from build123d import *

# Parameters (mm, degrees)
SKETCH1_R           = 6.35
BOSS_EXTRUDE1_DEPTH = 2.54
BOSS_EXTRUDE2_DEPTH = 12.7
SKETCH2_3_R         = 12.7
SKETCH2_3_R_2       = 6.35
BOSS_EXTRUDE3_DEPTH = 19.05
SKETCH2_5_R         = 6.35
BOSS_EXTRUDE4_DEPTH = 7.62
SKETCH5_R           = 6.35
CUT_EXTRUDE1_DEPTH  = 7.62


with BuildPart() as part:
    # Sketch1 → Boss-Extrude1 (new body)
    with BuildSketch(Plane(origin=(0, 0, 0), x_dir=(1, 0, 0), z_dir=(0, 1, 0))):
        with BuildLine():
            Line((12.7, 0), (63.5, 0))
            ThreePointArc((63.5, 0), (72.480256121, 3.719743879), (76.2, 12.7))
            Line((76.2, 12.7), (76.2, 50.8))
            ThreePointArc((76.2, 50.8), (72.480256121, 59.780256121), (63.5, 63.5))
            Line((63.5, 63.5), (12.7, 63.5))
            ThreePointArc((12.7, 63.5), (3.719743879, 59.780256121), (0, 50.8))
            Line((0, 50.8), (0, 12.7))
            ThreePointArc((0, 12.7), (3.719743879, 3.719743879), (12.7, 0))
        make_face()
        with Locations((12.7, 12.7)):
            Circle(SKETCH1_R, mode=Mode.SUBTRACT)
        with Locations((63.5, 12.7)):
            Circle(SKETCH1_R, mode=Mode.SUBTRACT)
    extrude(amount=BOSS_EXTRUDE1_DEPTH)

    # Sketch2 → Boss-Extrude2 (add)
    with BuildSketch(Plane(origin=(0, 2.54, 0), x_dir=(1, 0, 0), z_dir=(0, 1, 0))):
        with BuildLine():
            Line((63.5, 63.5), (12.7, 63.5))
            ThreePointArc((12.7, 63.5), (3.719743879, 59.780256121), (0, 50.8))
            ThreePointArc((0, 50.8), (0.544931264, 47.119741312), (2.132961262, 43.755307508))
            Line((2.132961262, 43.755307508), (27.532961262, 5.655307508))
            ThreePointArc((27.532961262, 5.655307508), (34.419741312, 24.855068736), (50.8, 12.7))
            ThreePointArc((50.8, 12.7), (50.255068736, 9.019741312), (48.667038738, 5.655307508))
            Line((48.667038738, 5.655307508), (74.067038738, 43.755307508))
            ThreePointArc((74.067038738, 43.755307508), (75.655068736, 47.119741312), (76.2, 50.8))
            ThreePointArc((76.2, 50.8), (72.480256121, 59.780256121), (63.5, 63.5))
        make_face()
        with BuildLine():
            Line((23.553103988, 16.204143539), (5.488594295, 43.300908078))
            ThreePointArc((5.488594295, 43.300908078), (4.924935684, 54.961088143), (14.939453481, 60.96))
            Line((14.939453481, 60.96), (61.260546519, 60.96))
            ThreePointArc((61.260546519, 60.96), (71.275064316, 54.961088143), (70.711405705, 43.300908078))
            Line((70.711405705, 43.300908078), (52.646896012, 16.204143539))
            ThreePointArc((52.646896012, 16.204143539), (38.1, 27.662994537), (23.553103988, 16.204143539))
        make_face(mode=Mode.SUBTRACT)
    extrude(amount=BOSS_EXTRUDE2_DEPTH)

    # Sketch2_3 → Boss-Extrude3 (add)
    with BuildSketch(Plane(origin=(0, 2.54, 0), x_dir=(1, 0, 0), z_dir=(0, 1, 0))):
        with Locations((38.1, 12.7)):
            Circle(SKETCH2_3_R)
        with Locations((38.1, 12.7)):
            Circle(SKETCH2_3_R_2, mode=Mode.SUBTRACT)
    extrude(amount=BOSS_EXTRUDE3_DEPTH)

    # Sketch2_5 → Boss-Extrude4 (add)
    with BuildSketch(Plane(origin=(0, 2.54, 0), x_dir=(1, 0, 0), z_dir=(0, 1, 0))):
        with BuildLine():
            ThreePointArc((61.260546519, 60.96), (71.275064316, 54.961088143), (70.711405705, 43.300908078))
            Line((70.711405705, 43.300908078), (52.646896012, 16.204143539))
            ThreePointArc((52.646896012, 16.204143539), (38.1, 27.662994537), (23.553103988, 16.204143539))
            Line((23.553103988, 16.204143539), (5.488594295, 43.300908078))
            ThreePointArc((5.488594295, 43.300908078), (4.924935684, 54.961088143), (14.939453481, 60.96))
            Line((14.939453481, 60.96), (61.260546519, 60.96))
        make_face()
        with Locations((63.5, 50.8)):
            Circle(SKETCH2_5_R, mode=Mode.SUBTRACT)
        with Locations((12.7, 50.8)):
            Circle(SKETCH2_5_R, mode=Mode.SUBTRACT)
    extrude(amount=BOSS_EXTRUDE4_DEPTH)

    # Sketch5 → Cut-Extrude1 (cut)
    with BuildSketch(Plane(origin=(0, 2.54, 0), x_dir=(1, 0, 0), z_dir=(0, 1, 0))):
        with Locations((12.7, 50.8)):
            Circle(SKETCH5_R)
        with Locations((63.5, 50.8)):
            Circle(SKETCH5_R)
        with Locations((38.1, 12.7)):
            Circle(SKETCH5_R)
    extrude(amount=-CUT_EXTRUDE1_DEPTH, mode=Mode.SUBTRACT)


solid = part.part
Check sheet for the modelled part. Datum: model origin and axes. Units: mm. A direction names the side the tool comes from. Round coordinates to 2 decimals unless told otherwise and drop trailing zeros. Order: outer loops, then holes, each group sorted by start corner. A loop starts at its lowest first (then second) coordinate and runs counter-clockwise, first axis right, second up.
(1) Scan lines: probe 1 along Z at (x, y) = (12.7, 1.7); probe 2 along X at (y, z) = (1.5, -50.8); probe 3 along X at (y, z) = (1.45, -12.7). Record each from-to range of solid material in increasing order.
(2) Cross-section at B-B, the plane x = 42. Enter the section's corners in (y, z), and give its area (3 significant figures).
(3) Access from +Z, -Z, +X, -X, +Y, -Y to the whole of each face (thin tool, end or side, straight path). Record for faces 4 (the flat face through (0, 1, -32)), 5 (the flat face through (14.655, 8.801, -24.972)), 6 (the cylindrical face through (3.62, 1.25, -3.82)), 7 (the flat face through (61.19, 8.8, -24.44)), 8 (the cylindrical face through (35.35, 14.05, -0.3)).
(4) Cross-section at A-A, the plane y = 4.75. Enter the section's corners in (x, z), and give its area (3 significant figures).
(5) Cross-section at D-D, the plane x = 59. Enter the section's corners in (y, z).
(6) Go/stop test with flat-tipped pins: P1, Ø3, axis at y = 18.5, z = -17, coming from the +X side; P2, Ø7.5, axis at x = 38.1, z = -12.7, coming from the +Y side; P3, Ø1.5, axis at x = 33.5, y = 13.5, coming from the +Z side; P4, Ø6, axis at x = 60, z = -52, coming from the +Y side. Record where each tip stops, or that it passes through.
(7) Draft check along X on faces 1 (the flat face through (76.2, 1, -31)), 2 (the flat face through (38, 15.24, -26)), 3 (the cylindrical face through (67, 1, -18)). Enter one of: pulls with the +X half, pulls with the -X half, needs draft (parallel to the pull), parting line crosses it, or undercut.
(8) Cross-section at C-C, the plane z = -10.5. Enter the section's corners in (x, y).
Check sheet entries:
1. probe 1: z = -63.5 to -57.15, -44.45 to -19.05, -6.35 to 0
1. probe 2: x = 0 to 6.35, 19.05 to 57.15, 69.85 to 76.2
1. probe 3: x = 0 to 6.35, 19.05 to 31.75, 44.45 to 57.15, 69.85 to 76.2
2. outline: (0, -63.5) - (15.24, -63.5) - (15.24, -60.96) - (10.16, -60.96) - (10.16, -27.15) - (15.24, -27.15) - (15.24, -24.79) - (21.59, -24.79) - (21.59, -17.71) - (0, -17.71) - close; (0, -7.69) - (21.59, -7.69) - (21.59, -0.61) - (2.54, -0.61) - (2.54, 0) - (0, 0) - close
2. area: 725 mm2
3. face 4: +Z, -Z, -X, +Y, -Y
3. face 5: +Z, -X, +Y
3. face 6: +Z, -X, +Y, -Y
3. face 7: +Z, +X, +Y
3. face 8: +Y
4. outline: (2.13, -43.76) arc R12.7 ccw to (12.7, -63.5) - (63.5, -63.5) arc R12.7 ccw to (74.07, -43.76) - (48.67, -5.66) arc R12.7 ccw to (27.53, -5.66) - close; hole circle Ø12.7 at (12.7, -50.8); hole circle Ø12.7 at (38.1, -12.7); hole circle Ø12.7 at (63.5, -50.8)
4. area: 2,900 mm2
5. outline: (0, -63.5) - (15.24, -63.5) - (15.24, -60.96) - (10.16, -60.96) - (10.16, -55.28) - (0, -55.28) - close; (0, -46.32) - (10.16, -46.32) - (10.16, -25.73) - (15.24, -25.73) - (15.24, -21.15) - (2.54, -21.15) - (2.54, -17.18) - (0, -17.18) - close; (0, -8.22) - (2.54, -8.22) - (2.54, 0) - (0, 0) - close
6. P1: stops at x = 50.49
6. P2: passes through
6. P3: stops at z = -0.6
6. P4: stops at y = 10.16
7. face 1: pulls with the +X half
7. face 2: needs draft
7. face 3: undercut
8. outline: (0.19, 0) - (6.74, 0) - (6.74, 2.54) - (0.19, 2.54) - close; (18.66, 0) - (32.14, 0) - (32.14, 21.59) - (25.59, 21.59) - (25.59, 15.24) - (24.3, 15.24) - (24.3, 2.54) - (18.66, 2.54) - close; (44.06, 0) - (57.54, 0) - (57.54, 2.54) - (51.9, 2.54) - (51.9, 15.24) - (50.61, 15.24) - (50.61, 21.59) - (44.06, 21.59) - close; (69.46, 0) - (76.01, 0) - (76.01, 2.54) - (69.46, 2.54) - close
